Check sheet for the modelled part. Datum: model origin and axes. Units: mm. Round coordinates to 2 decimals unless told otherwise and drop trailing zeros. Order: outer loops, then holes, each group sorted by start corner. A loop starts at its lowest first (then second) coordinate and runs counter-clockwise, first axis right, second up. Notation, with made-up numbers: (6, 35) -> (57, 35) arc R33 cw to (57, 71) -> close; hole circle Ø7 at (-14.5, 16.25). An arc over 180 degrees is marked (long way). Answer in a Markdown table with one row per item.
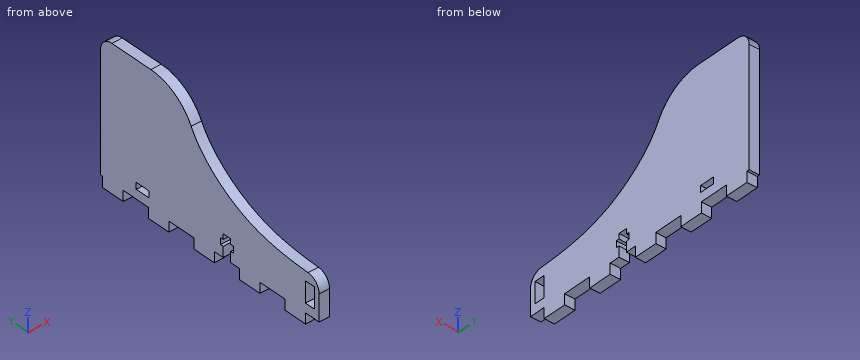
```python
from build123d import *

# Parameters (mm, degrees)
F0_W     = 4
F0_H     = 8
F0_W_2   = 5.6
F0_H_2   = 2.5
F1_DEPTH = 4
F2_R     = 20
F3_R     = 5


with BuildPart() as f1:
    # F0 (on Right) → F1 (new body)
    with BuildSketch(Plane.YZ):
        with BuildLine():
            Line((49, -4), (49, 0))
            Line((49, 0), (50, 0))
            Line((50, 0), (50, 50))
            Line((50, 50), (49, 50))
            Line((49, 50), (13, 50))
            add(Edge.make_bspline(
                [(13, 50), (12.9998758082, 38.0063697851), (-8.6775983117, 16.9623554105), (-32.0279580626, 15.0926403149), (-46, 15)],
                knots=[0, 0, 0, 0, 0.4916803973, 1, 1, 1, 1], degree=3))
            Line((-46, 15), (-46, 0))
            Line((-46, 0), (-40, 0))
            Line((-40, 0), (-40, -4))
            Line((-40, -4), (-31, -4))
            Line((-31, -4), (-31, 0))
            Line((-31, 0), (-20, 0))
            Line((-20, 0), (-20, -4))
            Line((-20, -4), (-11, -4))
            Line((-11, -4), (-11, 0))
            Line((-11, 0), (-7.15, 0))
            Line((-7.15, 0), (-7.15, 4))
            Line((-7.15, 4), (-8.3, 4))
            Line((-8.3, 4), (-8.3, 6.5))
            Line((-8.3, 6.5), (-7.15, 6.5))
            Line((-7.15, 6.5), (-7.15, 8.5))
            Line((-7.15, 8.5), (-5.5, 8.5))
            Line((-5.5, 8.5), (-3.85, 8.5))
            Line((-3.85, 8.5), (-3.85, 6.5))
            Line((-3.85, 6.5), (-2.7, 6.5))
            Line((-2.7, 6.5), (-2.7, 4))
            Line((-2.7, 4), (-3.85, 4))
            Line((-3.85, 4), (-3.85, 0))
            Line((-3.85, 0), (0, 0))
            Line((0, 0), (0, -4))
            Line((0, -4), (9, -4))
            Line((9, -4), (9, 0))
            Line((9, 0), (20, 0))
            Line((20, 0), (20, -4))
            Line((20, -4), (29, -4))
            Line((29, -4), (29, 0))
            Line((29, 0), (40, 0))
            Line((40, 0), (40, -4))
            Line((40, -4), (49, -4))
        make_face()
        with Locations((-42, 7.5)):
            Rectangle(F0_W, F0_H, mode=Mode.SUBTRACT)
        with Locations((31.5, 4.75)):
            Rectangle(F0_W_2, F0_H_2, mode=Mode.SUBTRACT)
    extrude(amount=F1_DEPTH)

    # F2
    f2_edges = [f1.edges().sort_by_distance(p)[0] for p in [
        (2, 13, 50),
    ]]
    fillet(f2_edges, radius=F2_R)

    # F3
    f3_edges = [f1.edges().sort_by_distance(p)[0] for p in [
        (2, 50, 50),
        (2, -46, 15),
    ]]
    fillet(f3_edges, radius=F3_R)


solid = f1.part
```
(1) Scan lines: probe 1 along Y at (x, z) = (0.55, 7); probe 2 along Z at (x, y) = (3.3, 30.5); probe 3 along Y at (x, z) = (3.05, 11). Record each from-to range of solid material in increasing order. Write a range as from..to.
Solutions:
| item | result |
|---|---|
| probe 1 | -46..-44, -40..-7.15, -3.85..50 |
| probe 2 | 0..3.5, 6..50 |
| probe 3 | -45.91..-44, -40..50 |
(2) Depth check by flat-ended pin: pin 1 Ø2 at (x, z) = (1, -2.5) entering from +Y; pin 2 Ø1.2 at (x, y) = (1, -41.5) entering from +Z; pin 3 Ø2 at (x, z) = (1.5, -2) entering from -Y. Enter the tip coordinate at first touch or a pass-through.
Solutions:
| item | result |
|---|---|
| pin 1 | y = 49 |
| pin 2 | z = 15.08 |
| pin 3 | y = -40 |
(3) Section check A-A on x = 1.2. Give the number of separate pieces and of enclosed holes in the cut face, plus the area to 3 significant figures.
Solutions:
| item | result |
|---|---|
| separate pieces | 1 |
| enclosed holes | 2 |
| area | 3,200 mm^2 |
(4) Section check B-B on y = 39. Record the boundary of the cut face in (x, z).
Solutions:
| item | result |
|---|---|
| outline | (0, 0) -> (4, 0) -> (4, 50) -> (0, 50) -> close |
